Design review of the part shown in the three views and the two pictorial views. Dimensions are in mm from the part's minimum x, y and z. A direction names the side the tool comes from. Give positions to 0.01 mm unless a question says otherwise; leave off trailing zeros. Write each loop counter-clockwise with the first axis right and the second up, starting at its lowest first coordinate (ties: lowest second). Pieces come first, ordered by that corner, then holes.
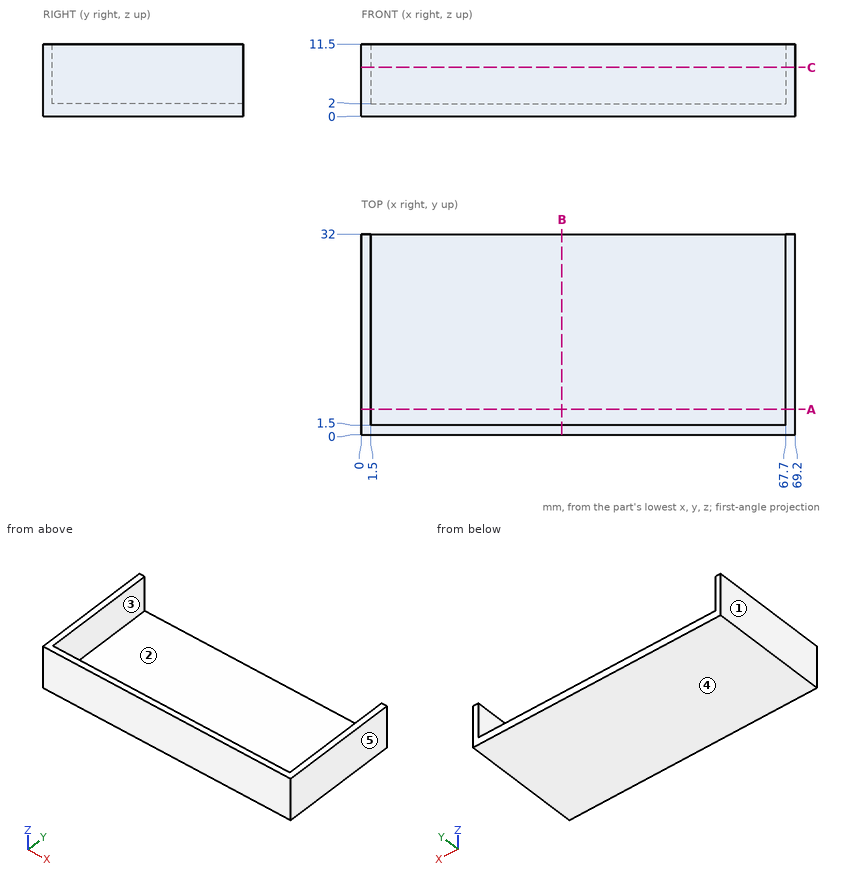
(1) Consider section B-B, the plane x = 32. Give the boundary of the cut face in (y, z), then the cut area to 4 significant figures.
Resolved:
outline: (0, 0) - (32, 0) - (32, 2) - (1.5, 2) - (1.5, 11.5) - (0, 11.5) - close
area: 78.25 mm2
(2) Tool access review of the marked faces 1 and 2: name each direction out of +Z, -Z, +X, -X, +Y, -Y from which nothing blocks a thin tool from reaching the whole face with its end or side.
Resolved:
face 1: +Z, -Z, -X, +Y, -Y
face 2: +Z, +Y
(3) Mouldability with a two-part tool opening along X and no side actions: class the marked faces 3, 4 and 5 as pulls with the +X half, pulls with the -X half, needs draft (parallel to the pull), parting line crosses it, or undercut.
Resolved:
face 3: undercut
face 4: needs draft
face 5: pulls with the +X half
(4) Clearance check with flat-ended pins moving along their axes: P1, Ø6, axis at x = 17, z = 10, coming from the +Y side; P2, Ø9, axis at x = 27.5, y = 10.5, coming from the +Z side; P3, Ø6, axis at x = 46.5, y = 22, coming from the -Z side. State where each tip first meets the part, or that it passes through.
Resolved:
P1: stops at y = 1.5
P2: stops at z = 2
P3: stops at z = 0
(5) Consider section A-A, the plane y = 4. Give the boundary of the cut face in (x, z), then the cut area to 3 significant figures.
Resolved:
outline: (0, 0) - (69.2, 0) - (69.2, 11.5) - (67.7, 11.5) - (67.7, 2) - (1.5, 2) - (1.5, 11.5) - (0, 11.5) - close
area: 167 mm2
(6) To check wall thickness, follow L1, parallel to X at y = 27.5, z = 9.75; L2, parallel to Y at x = 62, z = 4; L3, parallel to Z at x = 8, y = 23.5. State the ranges of each line that lie inside material, in increasing order.
Resolved:
L1: x = 0 to 1.5, 67.7 to 69.2
L2: y = 0 to 1.5
L3: z = 0 to 2
(7) Consider section C-C, the plane z = 7.75. Give the boundary of the cut face in (x, y), then the cut area to 3 significant figures.
Resolved:
outline: (0, 0) - (69.2, 0) - (69.2, 32) - (67.7, 32) - (67.7, 1.5) - (1.5, 1.5) - (1.5, 32) - (0, 32) - close
area: 195 mm2
